CAD build for the part. Positions are in the model's coordinates, mm. A direction names the side the tool comes from. Round coordinates to 2 decimals unless told otherwise and drop trailing zeros. Order: outer loops, then holes, each group sorted by start corner. A loop starts at its lowest first (then second) coordinate and runs counter-clockwise, first axis right, second up. Notation, with made-up numbers: M 88,8 L 114,8 A36 ccw 114,45 Z; hole C -13.5,62.5 d11. An arc over 180 degrees is marked long. Answer as a JSON object with one key per item and string values. Group by question number.
```python
from build123d import *

# Parameters (mm, degrees)
F1_DEPTH = 19.05
F3_DEPTH = 6.35
F4_W     = 19.05
F4_H     = 38.1
F5_DEPTH = 25.4
F6_W     = 63.5
F6_H     = 19.05
F7_DEPTH = 19.05


with BuildPart() as f1:
    # F0 (on Top) → F1 (new body)
    with BuildSketch(Plane.XY):
        Polygon((-486.346572, 384.430752), (-486.346572, -377.569248), (275.653428, -377.569248), align=None)
    extrude(amount=F1_DEPTH)

    # F2 (on face) → F3 (cut)
    with BuildSketch(Plane(origin=(0, 0, 0), x_dir=(1, 0, 0), z_dir=(0, 0, -1))):
        with BuildLine():
            ThreePointArc((-422.846572, 123.569248), (-435.546572, 136.269248), (-448.246572, 123.569248))
            Line((-448.246572, 123.569248), (-422.846572, 123.569248))
        make_face()
        with BuildLine():
            ThreePointArc((-16.446572, 123.569248), (-29.146572, 136.269248), (-41.846572, 123.569248))
            Line((-41.846572, 123.569248), (-16.446572, 123.569248))
        make_face()
        with BuildLine():
            Line((-16.446572, 123.569248), (-41.846572, 123.569248))
            ThreePointArc((-41.846572, 123.569248), (-29.146572, 110.869248), (-16.446572, 123.569248))
        make_face()
        with BuildLine():
            ThreePointArc((-67.246572, 123.569248), (-79.946572, 136.269248), (-92.646572, 123.569248))
            Line((-92.646572, 123.569248), (-67.246572, 123.569248))
        make_face()
        with BuildLine():
            Line((-67.246572, 123.569248), (-92.646572, 123.569248))
            ThreePointArc((-92.646572, 123.569248), (-79.946572, 110.869248), (-67.246572, 123.569248))
        make_face()
        with BuildLine():
            ThreePointArc((-118.046572, 123.569248), (-130.746572, 136.269248), (-143.446572, 123.569248))
            Line((-143.446572, 123.569248), (-118.046572, 123.569248))
        make_face()
        with BuildLine():
            Line((-118.046572, 123.569248), (-143.446572, 123.569248))
            ThreePointArc((-143.446572, 123.569248), (-130.746572, 110.869248), (-118.046572, 123.569248))
        make_face()
        with BuildLine():
            ThreePointArc((-168.846572, 123.569248), (-181.546572, 136.269248), (-194.246572, 123.569248))
            Line((-194.246572, 123.569248), (-168.846572, 123.569248))
        make_face()
        with BuildLine():
            Line((-168.846572, 123.569248), (-194.246572, 123.569248))
            ThreePointArc((-194.246572, 123.569248), (-181.546572, 110.869248), (-168.846572, 123.569248))
        make_face()
        with BuildLine():
            ThreePointArc((-219.646572, 123.569248), (-232.346572, 136.269248), (-245.046572, 123.569248))
            Line((-245.046572, 123.569248), (-219.646572, 123.569248))
        make_face()
        with BuildLine():
            Line((-219.646572, 123.569248), (-245.046572, 123.569248))
            ThreePointArc((-245.046572, 123.569248), (-232.346572, 110.869248), (-219.646572, 123.569248))
        make_face()
        with BuildLine():
            ThreePointArc((-270.446572, 123.569248), (-283.146572, 136.269248), (-295.846572, 123.569248))
            Line((-295.846572, 123.569248), (-270.446572, 123.569248))
        make_face()
        with BuildLine():
            Line((-270.446572, 123.569248), (-295.846572, 123.569248))
            ThreePointArc((-295.846572, 123.569248), (-283.146572, 110.869248), (-270.446572, 123.569248))
        make_face()
        with BuildLine():
            ThreePointArc((-321.246572, 123.569248), (-333.946572, 136.269248), (-346.646572, 123.569248))
            Line((-346.646572, 123.569248), (-321.246572, 123.569248))
        make_face()
        with BuildLine():
            Line((-321.246572, 123.569248), (-346.646572, 123.569248))
            ThreePointArc((-346.646572, 123.569248), (-333.946572, 110.869248), (-321.246572, 123.569248))
        make_face()
        with BuildLine():
            ThreePointArc((-372.046572, 123.569248), (-384.746572, 136.269248), (-397.446572, 123.569248))
            Line((-397.446572, 123.569248), (-372.046572, 123.569248))
        make_face()
        with BuildLine():
            Line((-372.046572, 123.569248), (-397.446572, 123.569248))
            ThreePointArc((-397.446572, 123.569248), (-384.746572, 110.869248), (-372.046572, 123.569248))
        make_face()
        with BuildLine():
            Line((-422.846572, 123.569248), (-448.246572, 123.569248))
            ThreePointArc((-448.246572, 123.569248), (-435.546572, 110.869248), (-422.846572, 123.569248))
        make_face()
        with BuildLine():
            ThreePointArc((-308.546572, -130.430752), (-295.846572, -143.130752), (-283.146572, -130.430752))
            Line((-283.146572, -130.430752), (-308.546572, -130.430752))
        make_face()
        with BuildLine():
            Line((-308.546572, -130.430752), (-283.146572, -130.430752))
            ThreePointArc((-283.146572, -130.430752), (-295.846572, -117.730752), (-308.546572, -130.430752))
        make_face()
        with BuildLine():
            ThreePointArc((-435.546572, -130.430752), (-422.846572, -143.130752), (-410.146572, -130.430752))
            Line((-410.146572, -130.430752), (-435.546572, -130.430752))
        make_face()
        with BuildLine():
            Line((-435.546572, -130.430752), (-410.146572, -130.430752))
            ThreePointArc((-410.146572, -130.430752), (-422.846572, -117.730752), (-435.546572, -130.430752))
        make_face()
        with BuildLine():
            ThreePointArc((-372.046572, -130.430752), (-359.346572, -143.130752), (-346.646572, -130.430752))
            Line((-346.646572, -130.430752), (-372.046572, -130.430752))
        make_face()
        with BuildLine():
            Line((-372.046572, -130.430752), (-346.646572, -130.430752))
            ThreePointArc((-346.646572, -130.430752), (-359.346572, -117.730752), (-372.046572, -130.430752))
        make_face()
    extrude(amount=-F3_DEPTH, mode=Mode.SUBTRACT)

    # F4 (on face) → F5 (cut)
    with BuildSketch(Plane.XY.offset(19.05)):
        with Locations((-457.771572, -282.319248)):
            Rectangle(F4_W, F4_H)
        with Locations((-457.771572, -180.719248)):
            Rectangle(F4_W, F4_H)
        with Locations((31.178428, -282.319248)):
            Rectangle(F4_W, F4_H)
        with Locations((31.178428, -180.719248)):
            Rectangle(F4_W, F4_H)
    extrude(amount=-F5_DEPTH, mode=Mode.SUBTRACT)

    # F6 (on face) → F7 (join)
    with BuildSketch(Plane(origin=(-486.346572, 0, 0), x_dir=(0, -1, 0), z_dir=(-1, 0, 0))):
        with Locations((-314.580752, 9.525)):
            Rectangle(F6_W, F6_H)
        with Locations((307.719248, 9.525)):
            Rectangle(F6_W, F6_H)
        with Locations((168.019248, 9.525)):
            Rectangle(F6_W, F6_H)
        with Locations((-174.880752, 9.525)):
            Rectangle(F6_W, F6_H)
    extrude(amount=F7_DEPTH)


solid = f1.part
```
Item 1: Two-plate mould, pull along X, no slides. Class faces 6 (the face through (-345.68, -128.43, 3.13)), 7 (the face through (-496, 346.331, 9)), 8 (the face through (-505.397, 315, 10)): +X half, -X half, draft (parallel to the pull), parting line (faces both ways), or undercut.
Item 2: Cut at A-A, the plane z = 13. Give the number of separate pieces and of enclosed holes in the cut face, and give its area (3 significant figures).
Item 3: Cut at B-B, the plane y = 98. Give the cut face in (x, z).
Item 4: 3-axis set-ups, long thin cutter, end or side, ignore diameter. For faces 1 (the face through (21.653, -181, 10)), 2 (the face through (-496, -199.769, 9)), 3 (the face through (-29, -124, 6.35)), 4 (the face through (-207, -76, 0)), 5 (the face through (-505.397, -307, 10)): which of +Z, -Z, +X, -X, +Y, -Y reach the whole face in a straight line?
Item 5: Drill centre lines: line 1 (X direction, y = 128.5, z = 5); line 2 (Y direction, x = -458, z = 13.75); line 3 (X direction, y = 125.5, z = 6.75). Where is each one in solid material? Low to high. Write a range as [from, to].
Item 6: Flat gauge pins, fed straight in: pin 1 Ø12.5 at (x, y) = (-295, 136) entering from -Z; pin 2 Ø5 at (x, z) = (45.5, 4) entering from +Y; pin 3 Ø1.5 at (x, z) = (-363.5, 17) entering from +Y. Where does each tip first touch, or does it go through?
Item 7: Cut at C-C, the plane y = 6.5. Give the cut face in (x, z).
Response values:
{
 "1": {"face 6": "undercut", "face 7": "draft", "face 8": "-X half"},
 "2": {"separate pieces": "1", "enclosed holes": "4", "area": "292,000 mm^2"},
 "3": {"outline": "M -486.35,0 L -199.92,0 L -199.92,19.05 L -486.35,19.05 Z"},
 "4": {"face 1": "+Z, -Z", "face 2": "+Z, -Z, -X", "face 3": "-Z", "face 4": "-Z, +X, -X, +Y, -Y", "face 5": "+Z, -Z, -X, +Y, -Y"},
 "5": {"line 1": "[-486.35, -435.4], [-410.29, -371.9], [-346.79, -308.4], [-283.29, -230.42]", "line 2": "[-377.57, -301.37], [-263.27, -199.77], [-161.67, 356.08]", "line 3": "[-486.35, -227.42]"},
 "6": {"pin 1": "z = 6.35", "pin 2": "y = -144.92", "pin 3": "y = 262.33"},
 "7": {"outline": "M -486.35,0 L -108.42,0 L -108.42,19.05 L -486.35,19.05 Z"}
}
